Build history of the part. All positions in model axes, mm. Face numbers are marked on the shaded views. A direction names the side the tool comes from. Round coordinates to 2 decimals unless told otherwise and drop trailing zeros. Write each loop counter-clockwise with the first axis right and the second up, starting at its lowest first coordinate (ties: lowest second). Pieces come first, ordered by that corner, then holes.
Item 1: 3-axis set-ups, long thin cutter, end or side, ignore diameter. For the marked faces 3, 4 and 5: which of +Z, -Z, +X, -X, +Y, -Y reach the whole face in a straight line?
Item 2: Band-saw the part on D-D, the plane y = 20. Write the cut outline in (x, z).
Item 3: Drop flat-ended pins along their axis: pin 1 Ø8.5 at (x, y) = (-25, -20) entering from -Z; pin 2 Ø9 at (x, y) = (2, 15) entering from -Z; pin 3 Ø0.6 at (y, z) = (18.5, 0.5) entering from -X; pin 4 Ø4 at (x, y) = (10, -16) entering from +Z. Give the stop position or say it passes through.
Item 4: Band-saw the part on C-C, the plane x = -25. Write the cut outline in (y, z), then the cut area to 3 significant figures.
Item 5: Band-saw the part on A-A, the plane x = -4.75. Write the cut outline in (y, z).
Item 6: Wall check: probe 1 along X at (y, z) = (20, 3.1); probe 2 along Y at (x, z) = (10, 4.95); probe 3 along X at (y, z) = (4, 4.35). Give the ranges that are in metal, low to high.
Item 7: Mould opens along Y. For the marked faces 1 and 2 say: +Y half, -Y half, draft (parallel to the pull), parting line (faces both ways), or undercut.
Item 8: Band-saw the part on B-B, the plane y = 4. Write the cut outline in (x, z).
Autodesk Inventor part; units mm, degrees
ref_plane "YZ Plane" through (0, 0, 0) normal (1, 0, 0) x (0, 1, 0)
ref_plane "XZ Plane" through (0, 0, 0) normal (0, 1, 0) x (-1, 0, 0)
ref_plane "XY Plane" through (0, 0, 0) normal (0, 0, 1) x (1, 0, 0)
sketch "スケッチ1" plane through (0, 0, 0) normal (0, 0, 1) x (1, 0, 0)
  line L0 (30, -26) -> (-30, -26)
  line L1 (-30, -26) -> (-30, 26)
  line L2 (-30, 26) -> (30, 26)
  line L3 (30, 26) -> (30, -26)
  line L4 (30, -26) -> (-30, 26) construction
  line L5 (-30, -26) -> (30, 26) construction
  point P0 (0, 0)
  dimension "d0" = 60
  dimension "d1" = 52
extrude "押し出し1" add sketch "スケッチ1" along normal blind 6
sketch "スケッチ2" plane through (0, 0, 6) normal (0, 0, 1) x (1, 0, 0)
  line L0 (25, -20) -> (-25, -20)
  line L1 (-25, -20) -> (-25, 20)
  line L2 (-25, 20) -> (25, 20)
  line L3 (25, 20) -> (25, -20)
  line L4 (25, -20) -> (-25, 20) construction
  line L5 (-25, -20) -> (25, 20) construction
  line L6 (-30, -26) -> (30, -26)
  point P0 (0, 0)
  point P1 (0, 0)
  point P2 (-25, -1)
  point P3 (25, -1)
  dimension "d4" = 50
  dimension "d5" = 40
  dimension "d6" = 6
hole "穴1" at (-25, -1, 6) at (25, -1, 6) at (25, 20, 6) at (-25, 20, 6) at (-25, -20, 6) at (25, -20, 6) direction (0, 0, -1) diameter 5.4 depth 8.8
sketch "スケッチ3" plane through (0, 0, 6) normal (0, 0, 1) x (1, 0, 0)
  line L0 (-10, -16) -> (10, -16)
  line L1 (10, -16) -> (10, 4)
  line L2 (10, 4) -> (-10, 4)
  line L3 (-10, 4) -> (-10, -16)
  line L4 (-10, -16) -> (10, 4) construction
  line L5 (10, -16) -> (-10, 4) construction
  line L6 (-30, -26) -> (30, -26)
  point P0 (0, 0)
  point P1 (0, -6)
  dimension "d14" = 20
  dimension "d15" = 20
  dimension "d16" = 10
hole "穴2" at (-10, -16, 6) at (-10, 4, 6) at (10, 4, 6) at (10, -16, 6) direction (0, 0, -1) diameter 3.3 depth 8.8 counterbore diameter 6.5 counterbore depth 4
sketch "スケッチ4" plane through (0, 0, 0) normal (0, 0, -1) x (-1, 0, 0)
  circle A0 centre (-10, 4) radius 1.65
  circle A1 centre (10, -16) radius 1.65
  circle A2 centre (10, 4) radius 1.65
  circle A3 centre (-10, -16) radius 1.65
  circle A4 centre (25, -20) radius 2.7
  circle A5 centre (-25, 20) radius 2.7
  circle A6 centre (25, -1) radius 2.7
  circle A7 centre (-25, -1) radius 2.7
  circle A8 centre (25, 20) radius 2.7
  circle A9 centre (-25, -20) radius 2.7
  line L0 (-30, -26) -> (-30, 26)
  line L1 (30, -26) -> (-30, -26)
  line L2 (30, 26) -> (30, -26)
  line L3 (-30, 26) -> (30, 26)
  line L4 (-30, 26) -> (30, 26)
  line L5 (-11, 26) -> (11, 26)
  line L6 (11, 26) -> (11, 8)
  line L7 (11, 8) -> (-11, 8)
  line L8 (-11, 8) -> (-11, 26)
  point P0 (0, 0)
  point P1 (11, 26)
  point P2 (-11, 26)
  dimension "d24" = 22
  dimension "d25" = 18
  dimension "d26" = 11
extrude "押し出し2" cut sketch "スケッチ4" against normal blind 2 contours L3 L6 L7 L8
chamfer "面取り1" distance 2 angle 45 4 edges at (-30, 26, 3) (-30, -26, 3) (30, -26, 3) (30, 26, 3)
fillet "フィレット1" radius 2 8 edges at (30, 24, 3) (28, 26, 3) (-28, 26, 3) (-30, 24, 3) (-30, -24, 3) (-28, -26, 3) (28, -26, 3) (30, -24, 3)
sketch "スケッチ5" plane through (0, 0, 2) normal (0, 0, -1) x (-1, 0, 0)
  line L0 (11, 26) -> (11, 8)
  line L1 (-11, 26) -> (11, 26)
  line L2 (-11, 8) -> (-11, 26)
  line L3 (11, 8) -> (-11, 8)
  point P0 (0, 0)
  point P1 (-4.75, 20)
  point P2 (4.75, 20)
  dimension "d33" = 9.5
  dimension "d34" = 4.75
  dimension "d35" = 6
hole "穴3" at (4.75, 20, 2) at (-4.75, 20, 2) direction (0, 0, 1) diameter 1.9 depth 8.8
fillet "フィレット2" radius 2 2 edges at (11, 8, 1) (-11, 8, 1)
chamfer "面取り2" distance 1 angle 45 33 edges at (19.0858, 26, 0) (27.9369, 25.8478, 0) (29, 25, 0) (29.8478, 23.9369, 0) (30, 0, 0) (29.8478, -23.9369, 0) (29, -25, 0) (27.9369, -25.8478, 0) (0, -26, 0) (-27.9369, -25.8478, 0) (-29, -25, 0) (-29.8478, -23.9369, 0) (-30, 0, 0) (-29.8478, 23.9369, 0) (-29, 25, 0) (-27.9369, 25.8478, 0) (-19.0858, 26, 0) (0, 26, 6) (-27.9369, 25.8478, 6) (-29, 25, 6) (-29.8478, 23.9369, 6) (-30, 0, 6) (-29.8478, -23.9369, 6) (-29, -25, 6) (-27.9369, -25.8478, 6) (0, -26, 6) (27.9369, -25.8478, 6) (29, -25, 6) (29.8478, -23.9369, 6) (30, 0, 6) (29.8478, 23.9369, 6) (29, 25, 6) (27.9369, 25.8478, 6)
properties part number "Diode_Laser_Mount"
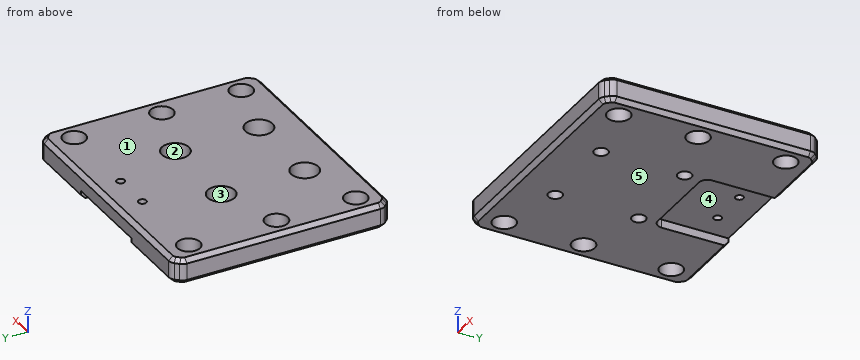
Results:
1. face 3: +Z
1. face 4: -Z, +Y
1. face 5: -Z, +X, -X, +Y, -Y
2. outline: (-30, 1) - (-29, 0) - (-27.7, 0) - (-27.7, 6) - (-29, 6) - (-30, 5) - close; (-22.3, 0) - (-11, 0) - (-11, 2) - (-5.7, 2) - (-5.7, 6) - (-22.3, 6) - close; (-3.8, 2) - (3.8, 2) - (3.8, 6) - (-3.8, 6) - close; (5.7, 2) - (11, 2) - (11, 0) - (22.3, 0) - (22.3, 6) - (5.7, 6) - close; (27.7, 0) - (29, 0) - (30, 1) - (30, 5) - (29, 6) - (27.7, 6) - close
3. pin 1: stops at z = 0
3. pin 2: stops at z = 2
3. pin 3: stops at x = -29.8
3. pin 4: stops at z = 2
4. outline: (-26, 1) - (-25, 0) - (-22.7, 0) - (-22.7, 6) - (-25, 6) - (-26, 5) - close; (-17.3, 0) - (-3.7, 0) - (-3.7, 6) - (-17.3, 6) - close; (1.7, 0) - (17.3, 0) - (17.3, 6) - (1.7, 6) - close; (22.7, 0) - (25, 0) - (26, 1) - (26, 5) - (25, 6) - (22.7, 6) - close
4. area: 213 mm2
5. outline: (-26, 1) - (-25, 0) - (8, 0) - (8, 2) - (19.05, 2) - (19.05, 6) - (-25, 6) - (-26, 5) - close; (20.95, 2) - (26, 2) - (26, 5) - (25, 6) - (20.95, 6) - close
6. probe 1: x = -30 to -27.7, -22.3 to -5.7, -3.8 to 3.8, 5.7 to 22.3, 27.7 to 30
6. probe 2: y = -26 to -19.25, -12.75 to 0.75, 7.25 to 26
6. probe 3: x = -30 to -13.25, -6.75 to 6.75, 13.25 to 30
7. face 1: draft
7. face 2: undercut
8. outline: (-30, 1) - (-29, 0) - (-11.65, 0) - (-11.65, 2) - (-13.25, 2) - (-13.25, 6) - (-29, 6) - (-30, 5) - close; (-8.35, 0) - (8.35, 0) - (8.35, 2) - (6.75, 2) - (6.75, 6) - (-6.75, 6) - (-6.75, 2) - (-8.35, 2) - close; (11.65, 0) - (29, 0) - (30, 1) - (30, 5) - (29, 6) - (13.25, 6) - (13.25, 2) - (11.65, 2) - close
